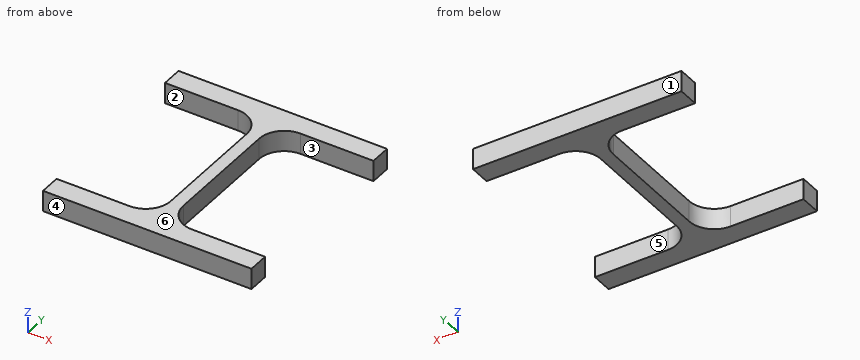
Autodesk Inventor part; units mm, degrees
ref_plane "YZ Plane" through (0, 0, 0) normal (1, 0, 0) x (0, 1, 0)
ref_plane "XZ Plane" through (0, 0, 0) normal (0, 1, 0) x (-1, 0, 0)
ref_plane "XY Plane" through (0, 0, 0) normal (0, 0, 1) x (1, 0, 0)
sketch "Блок1" plane through (0, 0, 0) normal (0, 0, 1) x (1, 0, 0)
  line L0 (-15, -40) -> (-50, -40)
  line L1 (-50, -40) -> (-50, -50)
  arc A0 (-15, -40) -> (-3, -28) centre (-15, -28) ccw
  arc A1 (3, -28) -> (15, -40) centre (15, -28) ccw
  line L2 (50, -40) -> (15, -40)
  line L3 (-50, -50) -> (50, -50)
  line L4 (15, 40) -> (50, 40)
  line L5 (50, 50) -> (-50, 50)
  line L6 (50, 40) -> (50, 50)
  line L7 (3, -28) -> (3, 28)
  line L8 (-3, 28) -> (-3, -28)
  line L9 (-50, 40) -> (-15, 40)
  arc A2 (-3, 28) -> (-15, 40) centre (-15, 28) ccw
  arc A3 (15, 40) -> (3, 28) centre (15, 28) ccw
  line L10 (-50, 50) -> (-50, 40)
  line L11 (50, -50) -> (50, -40)
  line L12 (-3, 0) -> (3, 0) construction
  point P0 (0, 0)
  point P1 (3, 40)
  point P2 (-3, 40)
  point P3 (0, 0)
  dimension "d12" = 100
  dimension "d13" = 100
  dimension "d14" = 6
  dimension "d15" = 10
  dimension "d16" = 12
sketch "Эскиз1" plane through (0, 0, 0) normal (0, 0, 1) x (1, 0, 0)
  line L0 (-3, 0) -> (3, 0) construction
  line L1 (-50, 40) -> (-15, 40)
  line L2 (-50, 50) -> (-50, 40)
  line L3 (50, 50) -> (-50, 50)
  line L4 (50, 40) -> (50, 50)
  line L5 (15, 40) -> (50, 40)
  line L6 (3, -28) -> (3, 28)
  line L7 (50, -40) -> (15, -40)
  line L8 (50, -50) -> (50, -40)
  line L9 (-50, -40) -> (-50, -50)
  line L10 (-15, -40) -> (-50, -40)
  line L11 (-3, 28) -> (-3, -28)
  arc A0 (-15, -40) -> (-3, -28) centre (-15, -28) ccw
  arc A1 (-3, 28) -> (-15, 40) centre (-15, 28) ccw
  arc A2 (15, 40) -> (3, 28) centre (15, 28) ccw
  arc A3 (3, -28) -> (15, -40) centre (15, -28) ccw
  line L12 (-50, -50) -> (50, -50)
  line L13 (0, 0) -> (0, 10) construction
  point P0 (-3, 40)
  point P1 (3, 40)
  dimension "d63" = 100
  dimension "d64" = 100
  dimension "d65" = 6
  dimension "d66" = 10
  dimension "d67" = 12
  dimension "d126" = 10
  dimension "d127" = 90
extrude "Выдавливание5" add sketch "Эскиз1" along normal blind 10
equation "\"d12\" = ParH"
equation "\"d13\" = b"
equation "\"d14\" = t1"
equation "\"d15\" = t2"
equation "\"d16\" = R1"
equation "\"d63\" = ParH"
equation "\"d64\" = b"
equation "\"d65\" = t1"
equation "\"d66\" = t2"
equation "\"d67\" = R1"
equation "\"ParH\" = 100"
equation "\"b\" = 100"
equation "\"t1\" = 6"
equation "\"t2\" = 10"
equation "\"R1\" = 12"
equation "\"Height\" = 96"
equation "\"Thickness1\" = 5"
equation "\"Thickness2\" = 8"
properties part number "IPB" material "Ст3сп ДСТУ 2651"
The listing builds one solid part. Answer for the finished solid, in the listing's coordinates (mm). Face numbers are marked on the shaded views. A direction names the side the tool comes from. Coordinates: 2 decimals unless noted, no trailing zeros. Loops run counter-clockwise (first coordinate to the right, second up) from the corner with the lowest first, then second, coordinate; pieces in that order, holes last.
1) Find section D-D on y = -11.5. Write down the section's boundary in (x, z), then the cut area to 3 significant figures.
2) A flat-ended cylindrical pin translates along its axis: pin 1 Ø2 at (y, z) = (-23.5, 2.5) entering from +X. Find the tip coordinate at first contact, or state that the pin passes through.
3) Find section A-A on x = -34. Write down the section's boundary in (y, z).
4) A tool of negligible diameter and unlimited length cuts with its end or side. For the marked faces 1, 2 and 3, from which of +Z, -Z, +X, -X, +Y, -Y can it reach the whole face along a straight path? Write none if from no direction.
5) Find the intervals of material crossed by L1, parallel to Y at x = 35.5, z = 2.5; L2, parallel to X at y = -28, z = 3.5; L3, parallel to Y at x = 9, z = 2.5, in increasing order.
6) Find section B-B on z = 1.75. Write down the section's boundary in (x, y), then the cut area to 3 significant figures.
7) Find section C-C on x = 6. Write down the section's boundary in (y, z), then the cut area to 3 significant figures.
8) Determine the mould class of the marked faces 4, 5 and 6 for opening direction Y: pulls with the +Y half, pulls with the -Y half, needs draft (parallel to the pull), parting line crosses it, or undercut.
Values:
1. outline: (-3, 0) - (3, 0) - (3, 10) - (-3, 10) - close
1. area: 60.0 mm2
2. pin 1: stops at x = 3
3. outline: (-50, 0) - (-40, 0) - (-40, 10) - (-50, 10) - close; (40, 0) - (50, 0) - (50, 10) - (40, 10) - close
4. face 1: +Z, -Z, +X, -X, +Y
4. face 2: +Z, -Z, -X
4. face 3: +Z, -Z, +X
5. L1: y = -50 to -40, 40 to 50
5. L2: x = -3 to 3
5. L3: y = -50 to -38.39, 38.39 to 50
6. outline: (-50, -50) - (50, -50) - (50, -40) - (15, -40) arc R12 cw to (3, -28) - (3, 28) arc R12 cw to (15, 40) - (50, 40) - (50, 50) - (-50, 50) - (-50, 40) - (-15, 40) arc R12 cw to (-3, 28) - (-3, -28) arc R12 cw to (-15, -40) - (-50, -40) - close
6. area: 2,600 mm2
7. outline: (-50, 0) - (-35.94, 0) - (-35.94, 10) - (-50, 10) - close; (35.94, 0) - (50, 0) - (50, 10) - (35.94, 10) - close
7. area: 281 mm2
8. face 4: pulls with the -Y half
8. face 5: undercut
8. face 6: needs draft
